from build123d import *

# Parameters (mm, degrees)
SCHIZZO3_R                   = 1.5
ESTRUSIONE_ESTRUSIONE2_DEPTH = 27.7
TAGLIO_ESTRUSIONE1_REACH     = 56.5
TAGLIO_ESTRUSIONE2_START     = -3
TAGLIO_ESTRUSIONE2_DEPTH     = 24.7


with BuildPart() as part:
    # Schizzo3 → Estrusione-Estrusione2 (new body)
    with BuildSketch(Plane(origin=(0, -1.8, 0), x_dir=(1, 0, 0), z_dir=(0, 1, 0))):
        with BuildLine():
            Line((27.25, -1.6), (27.25, -8.6))
            ThreePointArc((27.25, -8.6), (26.957106781, -9.307106781), (26.25, -9.6))
            Line((26.25, -9.6), (22.777350269, -9.6))
            ThreePointArc((22.777350269, -9.6), (22.277350269, -9.733974596), (21.911324865, -10.1))
            Line((21.911324865, -10.1), (20.872094381, -11.9))
            ThreePointArc((20.872094381, -11.9), (20.506068977, -12.266025404), (20.006068977, -12.4))
            Line((20.006068977, -12.4), (-20.006068977, -12.4))
            ThreePointArc((-20.006068977, -12.4), (-20.506068977, -12.266025404), (-20.872094381, -11.9))
            Line((-20.872094381, -11.9), (-21.911324865, -10.1))
            ThreePointArc((-21.911324865, -10.1), (-22.277350269, -9.733974596), (-22.777350269, -9.6))
            Line((-22.777350269, -9.6), (-26.25, -9.6))
            ThreePointArc((-26.25, -9.6), (-26.957106781, -9.307106781), (-27.25, -8.6))
            Line((-27.25, -8.6), (-27.25, -1.6))
            Line((-27.25, -1.6), (-27.25, 1.6))
            Line((-27.25, 1.6), (-27.25, 8.6))
            ThreePointArc((-27.25, 8.6), (-26.957106781, 9.307106781), (-26.25, 9.6))
            Line((-26.25, 9.6), (-22.777350269, 9.6))
            ThreePointArc((-22.777350269, 9.6), (-22.277350269, 9.733974596), (-21.911324865, 10.1))
            Line((-21.911324865, 10.1), (-20.872094381, 11.9))
            ThreePointArc((-20.872094381, 11.9), (-20.506068977, 12.266025404), (-20.006068977, 12.4))
            Line((-20.006068977, 12.4), (20.006068977, 12.4))
            ThreePointArc((20.006068977, 12.4), (20.506068977, 12.266025404), (20.872094381, 11.9))
            Line((20.872094381, 11.9), (21.911324865, 10.1))
            ThreePointArc((21.911324865, 10.1), (22.277350269, 9.733974596), (22.777350269, 9.6))
            Line((22.777350269, 9.6), (26.25, 9.6))
            ThreePointArc((26.25, 9.6), (26.957106781, 9.307106781), (27.25, 8.6))
            Line((27.25, 8.6), (27.25, 1.6))
            Line((27.25, 1.6), (27.25, -1.6))
        make_face()
        with Locations((24.2, -5)):
            Circle(SCHIZZO3_R, mode=Mode.SUBTRACT)
        with Locations((24.2, 5)):
            Circle(SCHIZZO3_R, mode=Mode.SUBTRACT)
        with Locations((-24.2, 5)):
            Circle(SCHIZZO3_R, mode=Mode.SUBTRACT)
        with Locations((-24.2, -5)):
            Circle(SCHIZZO3_R, mode=Mode.SUBTRACT)
        with BuildLine():
            Line((-19.2, -9.9), (19.2, -9.9))
            ThreePointArc((19.2, -9.9), (19.907106781, -9.607106781), (20.2, -8.9))
            Line((20.2, -8.9), (20.2, 8.9))
            ThreePointArc((20.2, 8.9), (19.907106781, 9.607106781), (19.2, 9.9))
            Line((19.2, 9.9), (-19.2, 9.9))
            ThreePointArc((-19.2, 9.9), (-19.907106781, 9.607106781), (-20.2, 8.9))
            Line((-20.2, 8.9), (-20.2, -8.9))
            ThreePointArc((-20.2, -8.9), (-19.907106781, -9.607106781), (-19.2, -9.9))
        make_face(mode=Mode.SUBTRACT)
    extrude(amount=-ESTRUSIONE_ESTRUSIONE2_DEPTH)

    # Schizzo4 → Taglio-Estrusione1 (cut, up to next)
    with BuildSketch(Plane(origin=(27.25, 0, 0), x_dir=(0, 0, -1), z_dir=(1, 0, 0)), mode=Mode.PRIVATE) as taglio_estrusione1_sk1:
        with BuildLine():
            Line((-3.710237866, -17.5387571), (3.710237866, -17.5387571))
            ThreePointArc((3.710237866, -17.5387571), (4.417344647, -17.831650319), (4.710237866, -18.5387571))
            Line((4.710237866, -18.5387571), (4.710237866, -23.4612429))
            ThreePointArc((4.710237866, -23.4612429), (4.417344647, -24.168349681), (3.710237866, -24.4612429))
            Line((3.710237866, -24.4612429), (-3.710237866, -24.4612429))
            ThreePointArc((-3.710237866, -24.4612429), (-4.417344647, -24.168349681), (-4.710237866, -23.4612429))
            Line((-4.710237866, -23.4612429), (-4.710237866, -18.5387571))
            ThreePointArc((-4.710237866, -18.5387571), (-4.417344647, -17.831650319), (-3.710237866, -17.5387571))
        make_face()
    taglio_estrusione1_tool1 = extrude(taglio_estrusione1_sk1.sketch, amount=-TAGLIO_ESTRUSIONE1_REACH, mode=Mode.PRIVATE) & part.part
    add(taglio_estrusione1_tool1.solids().sort_by_distance((27.25, -21, 0))[0], mode=Mode.SUBTRACT)

    # Schizzo5 → Taglio-Estrusione2 (cut)
    with BuildSketch(Plane(origin=(0, -1.8, 0), x_dir=(1, 0, 0), z_dir=(0, 1, 0)).offset(TAGLIO_ESTRUSIONE2_START)):
        Polygon((27.25, 8.6), (27.25, -8.6), (27.507432363, -11.370727038), (21.911324865, -11.370727038), (21.911324865, -9.6), (21.911324865, 9.6), (21.911324865, 11.665734377), (27.25, 11.503675338), align=None)
    taglio_estrusione2 = extrude(amount=-TAGLIO_ESTRUSIONE2_DEPTH, mode=Mode.SUBTRACT)

    # Specchia1: Taglio-Estrusione2 across plane
    add(taglio_estrusione2.mirror(Plane(origin=(0, 0, 0), x_dir=(0, 0, 1), z_dir=(1, 0, 0))), mode=Mode.SUBTRACT)


solid = part.part
Part model, mm, in its own coordinate system. A direction names the side the tool comes from. Coordinates: 2 decimals unless noted, no trailing zeros. Write each loop counter-clockwise with the first axis right and the second up, starting at its lowest first coordinate (ties: lowest second). Pieces come first, ordered by that corner, then holes. Notation, with made-up numbers: M 85,82.5 L 113,82.5 A16 cw 113,87.5 Z; hole C 82.5,14 d4. An arc over 180 degrees is marked long. Return JSON: item names as keys, results as strings.
1. Saw through at B-B, the plane z = -1.25. Write the cut outline in (x, y).
Determined:
{"outline": "M -27.25,-4.8 L -21.91,-4.8 L -21.91,-29.5 L -20.2,-29.5 L -20.2,-1.8 L -27.25,-1.8 Z; M 20.2,-29.5 L 21.91,-29.5 L 21.91,-24.46 L 20.2,-24.46 Z; M 20.2,-17.54 L 21.91,-17.54 L 21.91,-4.8 L 27.25,-4.8 L 27.25,-1.8 L 20.2,-1.8 Z"}
2. Flat gauge pins, fed straight in: pin 1 Ø1 at (y, z) = (-21.5, -4) entering from +X; pin 2 Ø2.5 at (x, y) = (24.5, -4) entering from +Z; pin 3 Ø1.5 at (y, z) = (-16, 2.5) entering from -X. Where does each tip first touch, or does it go through?
Determined:
{"pin 1": "x = -20.2", "pin 2": "z = 9.6", "pin 3": "x = -21.91"}
3. Pull direction Z, two halves, no side cores. Call faces 4 (the face through (25, -3, 9.6)), 5 (the face through (-22.77, -3.28, -5.45)), 6 (the face through (-27.25, -3, 0)), 7 (the face through (21.068, -24.176, 4.41)): pulls with the +Z half, pulls with the -Z half, needs draft (parallel to the pull), parting line crosses it, or undercut.
Determined:
{"face 4": "pulls with the +Z half", "face 5": "undercut", "face 6": "needs draft", "face 7": "undercut"}
4. Saw through at D-D, the plane x = -24.2. Write the cut outline in (y, z).
Determined:
{"outline": "M -4.8,-9.6 L -1.8,-9.6 L -1.8,-6.5 L -4.8,-6.5 Z; M -4.8,-3.5 L -1.8,-3.5 L -1.8,3.5 L -4.8,3.5 Z; M -4.8,6.5 L -1.8,6.5 L -1.8,9.6 L -4.8,9.6 Z"}
5. 3-axis set-ups, long thin cutter, end or side, ignore diameter. For faces 1 (the face through (-21.911, -17, 0)), 2 (the face through (0, -15, -9.9)), 3 (the face through (21.911, -17, 0)): which of +Z, -Z, +X, -X, +Y, -Y reach the whole face in a straight line?
Determined:
{"face 1": "+Z, -Z, -X, -Y", "face 2": "+Y, -Y", "face 3": "+Z, -Z, +X, -Y"}
6. Saw through at C-C, the plane y = -11.75. Write the cut outline in (x, z).
Determined:
{"outline": "M -21.91,-10.1 L -20.87,-11.9 A1 ccw -20.01,-12.4 L 20.01,-12.4 A1 ccw 20.87,-11.9 L 21.91,-10.1 L 21.91,10.1 L 20.87,11.9 A1 ccw 20.01,12.4 L -20.01,12.4 A1 ccw -20.87,11.9 L -21.91,10.1 Z; hole M -20.2,-8.9 A1 ccw -19.2,-9.9 L 19.2,-9.9 A1 ccw 20.2,-8.9 L 20.2,8.9 A1 ccw 19.2,9.9 L -19.2,9.9 A1 ccw -20.2,8.9 Z"}
7. Saw through at A-A, the plane x = -6. Write the cut outline in (y, z), then the cut area to 4 significant figures.
Determined:
{"outline": "M -29.5,-12.4 L -1.8,-12.4 L -1.8,-9.9 L -29.5,-9.9 Z; M -29.5,9.9 L -1.8,9.9 L -1.8,12.4 L -29.5,12.4 Z", "area": "138.5 mm²"}
8. Probe L1, parallel to Z at x = 24.2, y = -3.5; L2, parallel to X at y = -2.95, z = 5; L3, parallel to X at y = -18.5, z = -6.5. List the from-to ranges inside material, lowest first.
Determined:
{"L1": "-9.6 to -6.5, -3.5 to 3.5, 6.5 to 9.6", "L2": "-27.25 to -25.7, -22.7 to -20.2, 20.2 to 22.7, 25.7 to 27.25", "L3": "-21.91 to -20.2, 20.2 to 21.91"}
